```python
from build123d import *

# Parameters (mm, degrees)
SKETCH1_W           = 90.424
SKETCH1_H           = 84.074
BOSS_EXTRUDE1_DEPTH = 84.074
SKETCH3_W           = 85.344
SKETCH3_H           = 78.994
CUT_EXTRUDE1_DEPTH  = 81.534
SKETCH5_W           = 34.544
SKETCH5_H           = 10.414
CUT_EXTRUDE3_DEPTH  = 7.62
FILLET1_R           = 10.16
SKETCH6_W           = 9.652
SKETCH6_H           = 11.608529125
SKETCH6_W_2         = 12.446
SKETCH6_H_2         = 11.43
CUT_EXTRUDE4_DEPTH  = 5.08


with BuildPart() as part:
    # Sketch1 → Boss-Extrude1 (new body)
    with BuildSketch(Plane(origin=(0, 0, 0), x_dir=(1, 0, 0), z_dir=(0, 1, 0))):
        Rectangle(SKETCH1_W, SKETCH1_H)
    extrude(amount=BOSS_EXTRUDE1_DEPTH)

    # Sketch3 → Cut-Extrude1 (cut)
    with BuildSketch(Plane(origin=(0, 84.074, 0), x_dir=(1, 0, 0), z_dir=(0, 1, 0))):
        Rectangle(SKETCH3_W, SKETCH3_H)
    extrude(amount=-CUT_EXTRUDE1_DEPTH, mode=Mode.SUBTRACT)

    # Sketch5 → Cut-Extrude3 (cut)
    with BuildSketch(Plane.ZY.offset(45.212)):
        with Locations((0, 33.02)):
            Rectangle(SKETCH5_W, SKETCH5_H)
    extrude(amount=-CUT_EXTRUDE3_DEPTH, mode=Mode.SUBTRACT)

    # Fillet1
    fillet1_edges = [part.edges().sort_by_distance(p)[0] for p in [
        (42.672, 43.307, -39.497),
        (42.672, 43.307, 39.497),
        (-42.672, 43.307, 39.497),
        (-42.672, 43.307, -39.497),
        (45.212, 42.037, 42.037),
        (-45.212, 42.037, 42.037),
        (-45.212, 42.037, -42.037),
        (45.212, 42.037, -42.037),
    ]]
    fillet(fillet1_edges, radius=FILLET1_R)

    # Sketch6 → Cut-Extrude4 (cut)
    with BuildSketch(Plane(origin=(45.212, 0, 0), x_dir=(0, 0, -1), z_dir=(1, 0, 0))):
        with Locations((-18.477409208, 71.239969556)):
            Rectangle(SKETCH6_W, SKETCH6_H)
        with Locations((11.621294262, 71.24718083)):
            Rectangle(SKETCH6_W_2, SKETCH6_H_2)
    extrude(amount=-CUT_EXTRUDE4_DEPTH, mode=Mode.SUBTRACT)


solid = part.part
```
Could you check a few things on this model? Use its own coordinates, in mm. A direction names the side the tool comes from. Round coordinates to 2 decimals unless told otherwise and drop trailing zeros. Loops run counter-clockwise (first coordinate to the right, second up) from the corner with the lowest first, then second, coordinate; pieces in that order, holes last. Notation, with made-up numbers: M 54,11 L 82,11 A20 ccw 82,34 Z; hole C 1.25,80.5 d2. An arc over 180 degrees is marked long. Write item = value, one per line.
1. Which directions (+Z, -Z, +X, -X, +Y, -Y) give clear straight access to the entire face, cutting with the end or side of a thin tool? Please do faces 4 (the face through (-44, 33, 17.272)), 5 (the face through (44, 65.532, -12)), 6 (the face through (0, 44, -39.497)).
Results below:
face_4 = -X
face_5 = +X
face_6 = +Y
2. I want a section at D-D, the plane x = 3.5. Write out the boundary of the cut face in (y, z).
Results below:
outline = M 0,-42.04 L 84.07,-42.04 L 84.07,-39.5 L 2.54,-39.5 L 2.54,39.5 L 84.07,39.5 L 84.07,42.04 L 0,42.04 Z
3. I want a section at B-B, the plane z = -13. Write out the boundary of the cut face in (x, y).
Results below:
outline = M -45.21,0 L 45.21,0 L 45.21,65.53 L 42.67,65.53 L 42.67,2.54 L -42.67,2.54 L -42.67,27.81 L -45.21,27.81 Z; M -45.21,38.23 L -42.67,38.23 L -42.67,84.07 L -45.21,84.07 Z; M 42.67,76.96 L 45.21,76.96 L 45.21,84.07 L 42.67,84.07 Z
4. Will these pins go through, and if not, where does the flat tip stop? P1, Ø2, axis at x = 44.5, y = 74, coming from the +Z side; P2, Ø0.8, axis at x = 44.5, y = 73.5, coming from the +Z side; P3, Ø2, axis at x = 44, y = 72, coming from the -Z side.
Results below:
P1 = 37.52
P2 = 36.5
P3 = -38.21
5. I want a section at A-A, the plane y = 21.5. Write out the boundary of the cut face in (x, z).
Results below:
outline = M -45.21,-31.88 A10.16 ccw -35.05,-42.04 L 35.05,-42.04 A10.16 ccw 45.21,-31.88 L 45.21,31.88 A10.16 ccw 35.05,42.04 L -35.05,42.04 A10.16 ccw -45.21,31.88 Z; hole M -42.67,-29.34 A10.16 ccw -32.51,-39.5 L 32.51,-39.5 A10.16 ccw 42.67,-29.34 L 42.67,29.34 A10.16 ccw 32.51,39.5 L -32.51,39.5 A10.16 ccw -42.67,29.34 Z
6. I want a section at C-C, the plane z = -22. Write out the boundary of the cut face in (x, y).
Results below:
outline = M -45.21,0 L 45.21,0 L 45.21,84.07 L 42.67,84.07 L 42.67,2.54 L -42.67,2.54 L -42.67,84.07 L -45.21,84.07 Z
7. I need wall thicknesses on probe 1 along X at (y, z) = (61, -18); probe 2 along Z at (x, y) = (19, 5); probe 3 along X at (y, z) = (38, 38). Which ranges of each line are inside material? Lowest first, please.
Results below:
probe_1 = -45.21 to -42.67, 42.67 to 45.21
probe_2 = -42.04 to -39.5, 39.5 to 42.04
probe_3 = -43.16 to -37.82, 37.82 to 43.16
8. Thinking about a two-plate mould opening in Z: for faces 1 (the face through (0, 84.074, 40)), 2 (the face through (0, 44, 39.497)), 3 (the face through (-42.315, 42.626, -38.982)), which applies, +Z half, -Z half, draft (parallel to the pull), parting line (faces both ways), or undercut?
Results below:
face_1 = draft
face_2 = undercut
face_3 = -Z half
